Part model, mm, in its own coordinate system. Give positions to 0.01 mm unless a question says otherwise; leave off trailing zeros. Order: outer loops, then holes, each group sorted by start corner. A loop starts at its lowest first (then second) coordinate and runs counter-clockwise, first axis right, second up. Notation, with made-up numbers: (73, 67.5) - (110, 67.5) arc R15 cw to (110, 92.5) - close; hole circle Ø1 at (50, 20.5). An arc over 180 degrees is marked (long way). One line per item, written item: value.
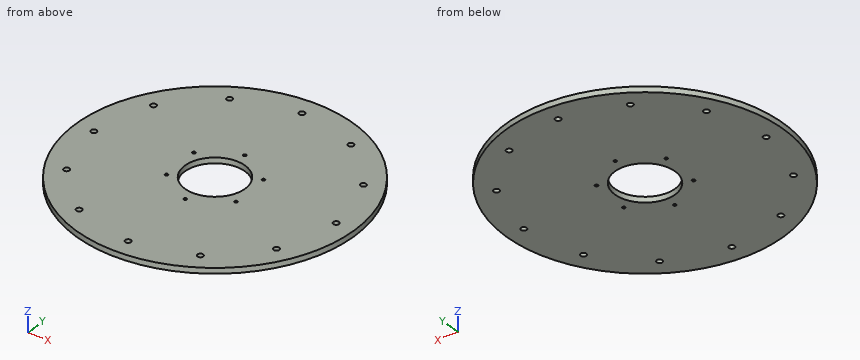
```python
from build123d import *

# Parameters (mm, degrees)
SKETCH_1_R      = 150
SKETCH_1_R_2    = 32.5
SKETCH_1_R_3    = 3.1
SKETCH_1_R_4    = 1.6
EXTRUDE_1_DEPTH = 6


with BuildPart() as part:
    # 草图1 → 凸台-拉伸1 (new body)
    with BuildSketch(Plane.XY):
        Circle(SKETCH_1_R)
        Circle(SKETCH_1_R_2, mode=Mode.SUBTRACT)
        with Locations((0, 130)):
            Circle(SKETCH_1_R_3, mode=Mode.SUBTRACT)
        with Locations((65, 112.583302492)):
            Circle(SKETCH_1_R_3, mode=Mode.SUBTRACT)
        with Locations((112.583302492, 65)):
            Circle(SKETCH_1_R_3, mode=Mode.SUBTRACT)
        with Locations((130, 0)):
            Circle(SKETCH_1_R_3, mode=Mode.SUBTRACT)
        with Locations((112.583302492, -65)):
            Circle(SKETCH_1_R_3, mode=Mode.SUBTRACT)
        with Locations((65, -112.583302492)):
            Circle(SKETCH_1_R_3, mode=Mode.SUBTRACT)
        with Locations((0, -130)):
            Circle(SKETCH_1_R_3, mode=Mode.SUBTRACT)
        with Locations((-65, -112.583302492)):
            Circle(SKETCH_1_R_3, mode=Mode.SUBTRACT)
        with Locations((-112.583302492, -65)):
            Circle(SKETCH_1_R_3, mode=Mode.SUBTRACT)
        with Locations((-130, 0)):
            Circle(SKETCH_1_R_3, mode=Mode.SUBTRACT)
        with Locations((-112.583302492, 65)):
            Circle(SKETCH_1_R_3, mode=Mode.SUBTRACT)
        with Locations((-65, 112.583302492)):
            Circle(SKETCH_1_R_3, mode=Mode.SUBTRACT)
        with Locations((0, 44.5)):
            Circle(SKETCH_1_R_4, mode=Mode.SUBTRACT)
        with Locations((38.538130468, -22.25)):
            Circle(SKETCH_1_R_4, mode=Mode.SUBTRACT)
        with Locations((0, -44.5)):
            Circle(SKETCH_1_R_4, mode=Mode.SUBTRACT)
        with Locations((-38.538130468, 22.25)):
            Circle(SKETCH_1_R_4, mode=Mode.SUBTRACT)
        with Locations((36.806829661, 21.250433013)):
            Circle(SKETCH_1_R_4, mode=Mode.SUBTRACT)
        with Locations(Location((-36.805329661, -21.249566987, 0), (0, 0, 180))):
            Circle(SKETCH_1_R_4, mode=Mode.SUBTRACT)
    extrude(amount=EXTRUDE_1_DEPTH)


solid = part.part
```
1) Cut at B-B, the plane z = 3.7. Give the number of separate pieces and of enclosed holes in the cut face, then the cut area to 3 significant figures.
Outcome:
separate pieces: 1
enclosed holes: 19
area: 67,000 mm^2
2) Drill centre lines: line 1 along Y through (x, z) = (0, 2.5); line 2 along X through (y, z) = (-130, 3.95); line 3 along Y through (x, z) = (28, 1.25). Where is each one in solid material? Low to high. Write a range as from..to.
Outcome:
line 1: y = -150..-133.1, -126.9..-46.1, -42.9..-32.5, 32.5..42.9, 46.1..126.9, 133.1..150
line 2: x = -74.83..-3.1, 3.1..74.83
line 3: y = -147.36..-16.5, 16.5..147.36
3) Cut at C-C, the plane y = -103.5. Give the cut face in (x, z).
Outcome:
outline: (-108.57, 0) - (108.57, 0) - (108.57, 6) - (-108.57, 6) - close
4) Cut at D-D, the plane x = 50. Give the cut face in (y, z).
Outcome:
outline: (-141.42, 0) - (141.42, 0) - (141.42, 6) - (-141.42, 6) - close
5) Cut at A-A, the plane x = 14.5. Give the cut face in (y, z), then the cut area to 3 significant figures.
Outcome:
outline: (-149.3, 0) - (-29.09, 0) - (-29.09, 6) - (-149.3, 6) - close; (29.09, 0) - (149.3, 0) - (149.3, 6) - (29.09, 6) - close
area: 1,440 mm^2
6) Pin check, flat tips, straight feed: pin 1 (2 mm diameter, centred on x = -97.5, z = 2.5, fed in from +Y); pin 2 (1.5 mm diameter, centred on y = 118.5, z = 5, fed in from -X); pin 3 (1 mm diameter, centred on x = 53, z = 2, fed in from -Y). Stop position of each tip, or through.
Outcome:
pin 1: stops at y = 114.84
pin 2: stops at x = -92.92
pin 3: stops at y = -140.51
